Verification items for the finished model (mm, model axes). A direction names the side the tool comes from. Give positions to 0.01 mm unless a question says otherwise; leave off trailing zeros. Loops run counter-clockwise (first coordinate to the right, second up) from the corner with the lowest first, then second, coordinate; pieces in that order, holes last. Notation, with made-up numbers: (72.25, 2) - (80.25, 2) arc R8 ccw to (80.25, 7) - close; hole circle Ø7 at (37, 84.25). An arc over 180 degrees is marked (long way). Use one line per item in the form item = value.
```python
from build123d import *

# Parameters (mm, degrees)
SKETCH1_W                    = 288.63
SKETCH1_H                    = 180
BOSS_EXTRUDE1_DEPTH          = 68
CUT_EXTRUDE5_DEPTH           = 69
BOSS_EXTRUDE2_DEPTH          = 15
BOSS_EXTRUDE3_DEPTH          = 15
SKETCH9_W                    = 44
SKETCH9_H                    = 180
CUT_EXTRUDE6_DEPTH           = 15
SKETCH10_W                   = 44
SKETCH10_H                   = 180
CUT_EXTRUDE7_DEPTH           = 15
M12_TAPPED_HOLE1_D           = 10.2
M12_TAPPED_HOLE1_DEPTH       = 98
M12_TAPPED_HOLE1_CSINK_D     = 12.05
M12_TAPPED_HOLE1_CSINK_ANGLE = 90
M12_TAPPED_HOLE2_D           = 10.2
M12_TAPPED_HOLE2_DEPTH       = 98
M12_TAPPED_HOLE2_CSINK_D     = 12.05
M12_TAPPED_HOLE2_CSINK_ANGLE = 90
M39_TAPPED_HOLE1_D           = 35
M39_TAPPED_HOLE1_DEPTH       = 25.484939167
M39_TAPPED_HOLE1_CSINK_D     = 39.05
M39_TAPPED_HOLE1_CSINK_ANGLE = 90
M39_TAPPED_HOLE1_TIP         = 10.515060833


with BuildPart() as part:
    # Sketch1 → Boss-Extrude1 (new body)
    with BuildSketch(Plane.XY):
        Rectangle(SKETCH1_W, SKETCH1_H)
    extrude(amount=BOSS_EXTRUDE1_DEPTH)

    # Sketch3 → Cut-Extrude5 (cut, through all)
    with BuildSketch(Plane.XY.offset(68)):
        Polygon((15, 15), (-15, 15), (-15, 0), (-30, 0), (-30, -15), (-45, -15), (-45, -30), (-60, -30), (-60, -45), (-75, -45), (-75, -60), (-90, -60), (-90, -75), (-105, -75), (-105, -90), (105, -90), (105, -75), (90, -75), (90, -60), (75, -60), (75, -45), (60, -45), (60, -30), (45, -30), (45, -15), (30, -15), (30, 0), (15, 0), align=None)
    extrude(amount=-CUT_EXTRUDE5_DEPTH, mode=Mode.SUBTRACT)

    # Sketch7 → Boss-Extrude2 (add)
    with BuildSketch(Plane.XY.offset(68)):
        with BuildLine():
            Line((-18, 90), (-18, 60))
            ThreePointArc((-18, 60), (0, 42), (18, 60))
            Line((18, 60), (18, 90))
            Line((18, 90), (-18, 90))
        make_face()
    extrude(amount=BOSS_EXTRUDE2_DEPTH)

    # Sketch8 → Boss-Extrude3 (add)
    with BuildSketch(Plane(origin=(0, 0, 0), x_dir=(-1, 0, 0), z_dir=(0, 0, -1))):
        with BuildLine():
            Line((-18, 90), (18, 90))
            Line((18, 90), (18, 60))
            ThreePointArc((18, 60), (0, 42), (-18, 60))
            Line((-18, 60), (-18, 90))
        make_face()
    extrude(amount=BOSS_EXTRUDE3_DEPTH)

    # Sketch9 → Cut-Extrude6 (cut)
    with BuildSketch(Plane.ZY.offset(144.315)):
        with Locations((34, 0)):
            Rectangle(SKETCH9_W, SKETCH9_H)
    extrude(amount=-CUT_EXTRUDE6_DEPTH, mode=Mode.SUBTRACT)

    # Sketch10 → Cut-Extrude7 (cut)
    with BuildSketch(Plane(origin=(144.315, 0, 0), x_dir=(0, 0, -1), z_dir=(1, 0, 0))):
        with Locations((-34, 0)):
            Rectangle(SKETCH10_W, SKETCH10_H)
    extrude(amount=-CUT_EXTRUDE7_DEPTH, mode=Mode.SUBTRACT)

    # M12 Tapped Hole1
    with Locations(Plane.XY.offset(83)):
        with Locations((0, 78)):
            CounterSinkHole(M12_TAPPED_HOLE1_D / 2, M12_TAPPED_HOLE1_CSINK_D / 2, depth=M12_TAPPED_HOLE1_DEPTH, counter_sink_angle=M12_TAPPED_HOLE1_CSINK_ANGLE)

    # M12 Tapped Hole2
    with Locations(Plane(origin=(0, 0, -15), x_dir=(-1, 0, 0), z_dir=(0, 0, -1))):
        with Locations((0, 78)):
            CounterSinkHole(M12_TAPPED_HOLE2_D / 2, M12_TAPPED_HOLE2_CSINK_D / 2, depth=M12_TAPPED_HOLE2_DEPTH, counter_sink_angle=M12_TAPPED_HOLE2_CSINK_ANGLE)

    # M39 Tapped Hole1
    with Locations(Plane(origin=(0, 90, 0), x_dir=(1, 0, 0), z_dir=(0, 1, 0))):
        with Locations((0, -34)):
            CounterSinkHole(M39_TAPPED_HOLE1_D / 2, M39_TAPPED_HOLE1_CSINK_D / 2, depth=M39_TAPPED_HOLE1_DEPTH, counter_sink_angle=M39_TAPPED_HOLE1_CSINK_ANGLE)
            with Locations((0, 0, -(M39_TAPPED_HOLE1_DEPTH + M39_TAPPED_HOLE1_TIP / 2))):  # 118° drill point
                Cone(0, M39_TAPPED_HOLE1_D / 2, M39_TAPPED_HOLE1_TIP, mode=Mode.SUBTRACT)


solid = part.part
```
1. Section check A-A, the plane y = -35. Record the cut outline in (x, z) (3 decimals).
Result set:
outline = (-144.315, 0) - (-60, 0) - (-60, 68) - (-144.315, 68) - (-144.315, 56) - (-129.315, 56) - (-129.315, 12) - (-144.315, 12) - close; (60, 0) - (144.315, 0) - (144.315, 12) - (129.315, 12) - (129.315, 56) - (144.315, 56) - (144.315, 68) - (60, 68) - close
2. Draft check along Z on faces 1 (the flat face through (-2, 21, 68)), 2 (the cylindrical face through (-16.166, 76.081, 40.703)), 3 (the flat face through (-45, -22, 34)). Enter one of: released by +Z, released by -Z, zero draft, split by the parting line, or undercut.
Result set:
face_1 = released by +Z
face_2 = undercut
face_3 = zero draft
3. Tool access check on faces 4 (the cylindrical face through (0, 42, -7)), 5 (the flat face through (53, -30, 34)), 6 (the flat face through (144.315, -1, 62)), 7 (the flat face through (129.315, 1, 34)). Record the directions out of +Z, -Z, +X, -X, +Y, -Y that give a thin tool (end or side, any length) a straight path to the whole face; none if there is none.
Result set:
face_4 = -Z, -Y
face_5 = +Z, -Z, -Y
face_6 = +Z, -Z, +X, +Y, -Y
face_7 = +X, +Y, -Y
4. Scan lines: probe 1 along X at (y, z) = (78, 10) (3 decimals); probe 2 along Y at (x, z) = (0, 1); probe 3 along X at (y, z) = (-30.5, 67) (3 decimals). Record each from-to range of solid material in increasing order.
Result set:
probe_1 = -144.315 to -5.1, 5.1 to 144.315
probe_2 = 15 to 72.9, 83.1 to 90
probe_3 = -144.315 to -60, 60 to 144.315
5. Section check B-B, the plane y = -55.5. Record the cut outline in (x, z) (3 decimals), then the cut area to 3 significant figures.
Result set:
outline = (-144.315, 0) - (-75, 0) - (-75, 68) - (-144.315, 68) - (-144.315, 56) - (-129.315, 56) - (-129.315, 12) - (-144.315, 12) - close; (75, 0) - (144.315, 0) - (144.315, 12) - (129.315, 12) - (129.315, 56) - (144.315, 56) - (144.315, 68) - (75, 68) - close
area = 8,110 mm²
6. Depth check by flat-ended pin: pin 1 Ø1.5 at (x, y) = (40.5, 14.5) entering from -Z; pin 2 Ø3 at (x, z) = (-91.5, 26) entering from -Y; pin 3 Ø4.5 at (y, z) = (-24.5, 23) entering from -X (3 decimals). Enter the tip coordinate at first touch or a pass-through.
Result set:
pin_1 = 0
pin_2 = -75
pin_3 = -129.315
